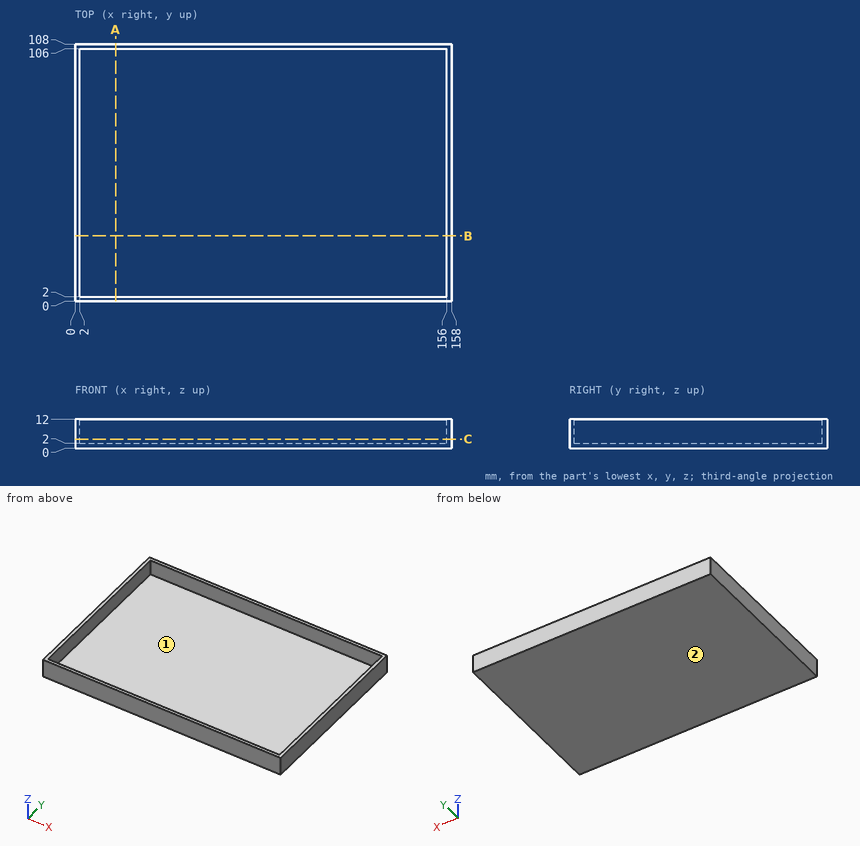
Geometry: see drawing. Coordinates: mm, zero at the bounding-box minimum. Round coordinates to 2 decimals unless told otherwise and drop trailing zeros. Write each loop counter-clockwise with the first axis right and the second up, starting at its lowest first coordinate (ties: lowest second). Pieces come first, ordered by that corner, then holes. Notation, with made-up numbers: (37, -15.5) - (45, -15.5) arc R34 ccw to (45, 15.5) - close; hole circle Ø4 at (-37, -38). An arc over 180 degrees is marked (long way). Use CSV: the item, a comma, the result in double quotes. Start each with the question number.
(1) Cut plane C-C, the plane z = 3.75. Return loops of the section in (x, y).
(2) Cut plane A-A, the plane x = 17. Return loops of the section in (y, z).
(3) Cut plane B-B, the plane y = 27.5. Return loops of the section in (x, z), and give its area (3 significant figures).
(4) Material intervals for probe 1 along X at (y, z) = (51.5, 7.25); probe 2 along Y at (x, z) = (122, 5); probe 3 along Z at (x, y) = (139, 53.5), sorted ascending. Write a range as [from, to].
(5) Mould query, pull axis X, two halves, no side actions, for the marked faces 1 and 2. Classes: pulls with the +X half, pulls with the -X half, needs draft (parallel to the pull), parting line crosses it, or undercut.
(6) First-contact query: pin 1 Ø1 at (x, y) = (139, 37.5) entering from +Z. Flat tip, straight axial feed; report the tip coordinate or a pass-through.
Geometry says:
1,outline,"(0, 0) - (158, 0) - (158, 108) - (0, 108) - close; hole (2, 2) - (156, 2) - (156, 106) - (2, 106) - close"
2,outline,"(0, 0) - (108, 0) - (108, 12) - (106, 12) - (106, 2) - (2, 2) - (2, 12) - (0, 12) - close"
3,outline,"(0, 0) - (158, 0) - (158, 12) - (156, 12) - (156, 2) - (2, 2) - (2, 12) - (0, 12) - close"
3,area,"356 mm²"
4,probe 1,"[0, 2], [156, 158]"
4,probe 2,"[0, 2], [106, 108]"
4,probe 3,"[0, 2]"
5,face 1,"undercut"
5,face 2,"needs draft"
6,pin 1,"z = 2"
